from build123d import *

# Parameters (mm, degrees)
EXTRUDE1_DEPTH = 2540
EXTRUDE2_START = 88.9
SKETCH2_W      = 406.11851991
SKETCH2_H      = 123.339698639
SKETCH2_H_2    = 529.458218549
EXTRUDE2_DEPTH = 2690.004184222


with BuildPart() as part:
    # Sketch1 → Extrude1 (new body)
    with BuildSketch(Plane(origin=(0, 0, 0), x_dir=(0, 1, 0), z_dir=(0, 0, 1))):
        Polygon((-379.260815056, -1250.091692764), (-356.400815056, -1250.091692764), (-356.400815056, -1274.700151443), (-432.600815056, -1274.700151443), (-432.600815056, -1250.091692764), (-409.740815056, -1250.091692764), (-409.740815056, -1225.483234085), (-432.600815056, -1225.483234085), (-477.441999719, -1225.483234085), (-477.441999719, -1274.700151443), (-553.641999719, -1274.700151443), (-553.641999719, -1183.595391403), (462.358000281, -1183.595391403), (462.358000281, -1274.700151443), (386.158000281, -1274.700151443), (386.158000281, -1225.483234085), (341.316815619, -1225.483234085), (318.456815619, -1225.483234085), (318.456815619, -1250.091692764), (341.316815619, -1250.091692764), (341.316815619, -1274.700151443), (265.116815619, -1274.700151443), (265.116815619, -1250.091692764), (287.976815619, -1250.091692764), (287.976815619, -1225.483234085), (265.116815619, -1225.483234085), (-356.400815056, -1225.483234085), (-379.260815056, -1225.483234085), align=None)
    extrude(amount=EXTRUDE1_DEPTH)

    # Sketch2 → Extrude2 (cut, through all)
    with BuildSketch(Plane(origin=(1225.483234085, 0, 0), x_dir=(0, 0, -1), z_dir=(1, 0, 0)).offset(EXTRUDE2_START)):
        with Locations((-1790.833583772, -456.272947628)):
            Rectangle(SKETCH2_W, SKETCH2_H)
        with Locations((-2298.833583772, -456.272947628)):
            Rectangle(SKETCH2_W, SKETCH2_H)
        with Locations((-2298.833583772, -45.641999719)):
            Rectangle(SKETCH2_W, SKETCH2_H_2)
        with Locations((-2298.833583772, 364.98894819)):
            Rectangle(SKETCH2_W, SKETCH2_H)
        with Locations((-1790.833583772, -45.641999719)):
            Rectangle(SKETCH2_W, SKETCH2_H_2)
        with Locations((-1790.833583772, 364.98894819)):
            Rectangle(SKETCH2_W, SKETCH2_H)
        with Locations((-1282.833583772, -456.272947628)):
            Rectangle(SKETCH2_W, SKETCH2_H)
        with Locations((-1282.833583772, -45.641999719)):
            Rectangle(SKETCH2_W, SKETCH2_H_2)
        with Locations((-1282.833583772, 364.98894819)):
            Rectangle(SKETCH2_W, SKETCH2_H)
        with Locations((-774.833583772, -456.272947628)):
            Rectangle(SKETCH2_W, SKETCH2_H)
        with Locations((-774.833583772, -45.641999719)):
            Rectangle(SKETCH2_W, SKETCH2_H_2)
        with Locations((-774.833583772, 364.98894819)):
            Rectangle(SKETCH2_W, SKETCH2_H)
        with Locations((-266.833583772, -456.272947628)):
            Rectangle(SKETCH2_W, SKETCH2_H)
        with Locations((-266.833583772, -45.641999719)):
            Rectangle(SKETCH2_W, SKETCH2_H_2)
        with Locations((-266.833583772, 364.98894819)):
            Rectangle(SKETCH2_W, SKETCH2_H)
    extrude(amount=-EXTRUDE2_DEPTH, mode=Mode.SUBTRACT)


solid = part.part
For this review, take the finished solid that the model builds, in its own axes (mm). A direction names the side the tool comes from. Give positions to 0.01 mm unless a question says otherwise; leave off trailing zeros. Order: outer loops, then holes, each group sorted by start corner. A loop starts at its lowest first (then second) coordinate and runs counter-clockwise, first axis right, second up. Notation, with made-up numbers: M 52,63.5 L 62,63.5 A25 ccw 62,77.5 Z; hole C -7.75,-8 d1. An arc over 180 degrees is marked long. Answer in a Markdown table with one row per item. Add a question column.
(1) For pin 1 (20.5 mm diameter, centred on y = -460, z = 1548.5, fed in from +X), flat-tipped, find the tip position at first contact; note if it passes through.
(2) Consider section D-D on x = 1209. Give the number of separate pieces and of enclosed holes in the cut face, and give its area (3 significant figures).
(3) Consider section A-A on y = -268. State the section outline as (x, z) points, and give its area (3 significant figures).
(4) Consider section C-C on z = 1536. State the section outline as (x, y) points, and give its area (3 significant figures).
(5) For faces 1 (the face through (1250, 386.158, 31)), 2 (the face through (1225.483, -121, 1076)), 3 (the face through (1230, 426.659, 778)), list the 3-axis set-ups (+Z, -Z, +X, -X, +Y, -Y) from which the entire face can be reached by the end or side of a thin tool; tool diameter is ignored.
(6) Consider section B-B on z = 2129. State the section outline as (x, y) points.
(7) Wall thickness on probe 1 along Z at (x, y) = (1217, -503); probe 2 along Y at (x, z) = (1263.5, 316.5); probe 3 along Y at (x, z) = (1190.5, 1871): over which ranges is each line inside the solid? List them lowest first. Write a range as [from, to].
Evaluation:
| question | item | result |
|---|---|---|
| 1 | pin 1 | stops at x = 1225.48 |
| 2 | separate pieces | 1 |
| 2 | enclosed holes | 15 |
| 2 | area | 1,000,000 mm^2 |
| 3 | outline | M 1183.6,0 L 1225.48,0 L 1225.48,63.77 L 1183.6,63.77 Z; M 1183.6,469.89 L 1225.48,469.89 L 1225.48,571.77 L 1183.6,571.77 Z; M 1183.6,977.89 L 1225.48,977.89 L 1225.48,1079.77 L 1183.6,1079.77 Z; M 1183.6,1485.89 L 1225.48,1485.89 L 1225.48,1587.77 L 1183.6,1587.77 Z; M 1183.6,1993.89 L 1225.48,1993.89 L 1225.48,2095.77 L 1183.6,2095.77 Z; M 1183.6,2501.89 L 1225.48,2501.89 L 1225.48,2540 L 1183.6,2540 Z |
| 3 | area | 21,300 mm^2 |
| 4 | outline | M 1183.6,-553.64 L 1274.7,-553.64 L 1274.7,-477.44 L 1225.48,-477.44 L 1225.48,-409.74 L 1250.09,-409.74 L 1250.09,-432.6 L 1274.7,-432.6 L 1274.7,-356.4 L 1250.09,-356.4 L 1250.09,-379.26 L 1225.48,-379.26 L 1225.48,287.98 L 1250.09,287.98 L 1250.09,265.12 L 1274.7,265.12 L 1274.7,341.32 L 1250.09,341.32 L 1250.09,318.46 L 1225.48,318.46 L 1225.48,386.16 L 1274.7,386.16 L 1274.7,462.36 L 1183.6,462.36 Z |
| 4 | area | 55,300 mm^2 |
| 5 | face 1 | +Z, -Z, +X |
| 5 | face 2 | +Z, -Z |
| 5 | face 3 | +X, -X |
| 6 | outline | M 1183.6,-553.64 L 1274.7,-553.64 L 1274.7,-517.94 L 1183.6,-517.94 Z; M 1183.6,-394.6 L 1274.7,-394.6 L 1274.7,-356.4 L 1250.09,-356.4 L 1250.09,-379.26 L 1225.48,-379.26 L 1225.48,-310.37 L 1183.6,-310.37 Z; M 1183.6,219.09 L 1225.48,219.09 L 1225.48,287.98 L 1250.09,287.98 L 1250.09,265.12 L 1274.7,265.12 L 1274.7,303.32 L 1183.6,303.32 Z; M 1183.6,426.66 L 1274.7,426.66 L 1274.7,462.36 L 1183.6,462.36 Z |
| 7 | probe 1 | z = [0, 63.77], [469.89, 571.77], [977.89, 1079.77], [1485.89, 1587.77], [1993.89, 2095.77], [2501.89, 2540] |
| 7 | probe 2 | y = [-553.64, -517.94], [-394.6, -356.4], [265.12, 303.32], [426.66, 462.36] |
| 7 | probe 3 | y = [-553.64, -517.94], [-394.6, -310.37], [219.09, 303.32], [426.66, 462.36] |
